```python
from build123d import *

# Parameters (mm, degrees)
F3_R = 0.99999


# Not quite as in the source:
# - a fillet or chamfer that OpenCascade refuses, or shapes differently, is made with other operations: its cross-section is extruded or revolved along the edge and cut away or added
# - a fillet or chamfer is up to 0.001 mm smaller than in the source, because OpenCascade refuses the exact size


with BuildPart() as f1:
    # F0 (on Right) → F1 (revolve)
    with BuildSketch(Plane.YZ):
        Polygon((-47.0208749175, 2.497), (-35.0208749175, 2.497), (-35.0208749175, 4.55), (-41.0208749175, 4.55), (-41.0208749175, 7.5), (-42.0208749175, 7.5), (-43.0208749175, 4.55), (-43.5208749175, 4.55), (-44.0208749175, 4.55), (-45.0208749175, 7.5), (-46.0208749175, 7.5), (-46.0208749175, 4.55), (-46.0208749175, 3.497), (-47.0208749175, 3.497), align=None)
    revolve(axis=Axis((0, -14.7727020085, 0), (0, 1, 0)))

    # F2: fillet of radius 5 on 1 edges, made by hand

    # F2_s1 → F2_t2 (revolve)
    with BuildSketch(Plane.YZ):
        with BuildLine():
            ThreePointArc((-36.460447306, 4.55), (-39.1761424288, 5.3517860941), (-41.0208749175, 7.5))
            Line((-41.0208749175, 7.5), (-41.1120834697, 7.459))
            ThreePointArc((-41.1120834697, 7.459), (-41.1208749175, 6.025), (-41.1208749175, 4.55))
            Line((-41.1208749175, 4.55), (-41.0208749175, 4.45))
            Line((-41.0208749175, 4.45), (-36.460447306, 4.45))
            Line((-36.460447306, 4.45), (-36.460447306, 4.55))
        make_face()
    revolve(axis=Axis((0, -41.0208749175, 0), (0, 1, 0)))

    # F3 (radius 1 in the source; OpenCascade refuses exactly that, so slightly less here)
    f3_edges = [f1.edges().sort_by_distance(p)[0] for p in [
        (0, -46.020875, -3.497),
    ]]
    fillet(f3_edges, radius=F3_R)


solid = f1.part
```
Model file for the job. Use its own axes, mm. A direction names the side the tool comes from. Round coordinates to 2 decimals unless told otherwise and drop trailing zeros. Write each loop counter-clockwise with the first axis right and the second up, starting at its lowest first coordinate (ties: lowest second). Pieces come first, ordered by that corner, then holes. Notation, with made-up numbers: (-38.75, 13) - (-4.75, 13) arc R25 ccw to (-4.75, 41) - close; hole circle Ø11 at (29, 16). An arc over 180 degrees is marked (long way). Use CSV: the item, a comma, the result in double quotes. Start each with the question number.
Item 1: Pin check, flat tips, straight feed: P1, Ø5, axis at x = 3, y = -41.5, coming from the -Z side; P2, Ø4, axis at x = -1, y = -38, coming from the +Z side; P3, Ø4, axis at x = -0.5, y = -41, coming from the +Z side. Stop position of each tip, or through.
Item 2: Tool access for faces 1 (the face through (-5, -46.021, 0)), 2 (the face through (-4.44, -43.53, -0.99)), 3 (the face through (-4.44, -35.75, -0.99)): list every direction of +Z, -Z, +X, -X, +Y, -Y with a clear straight run to the whole face (end or side of a thin tool).
Item 3: Drill centre lines: L1, parallel to X at y = -43.5, z = 0; L2, parallel to X at y = -41.75, z = 0; L3, parallel to X at y = -45.5, z = -6. Where is each one in solid material? Low to high. Write a range as [from, to].
Item 4: Band-saw the part on C-C (y = -41.75). Write the cut outline in (x, z).
Item 5: Band-saw the part on D-D (y = -36). Write the cut outline in (x, z), and give its area (3 significant figures).
Item 6: Two-plate mould, pull along Y, no slides. Class faces 4 (the face through (4.694, -44.083, -0.616)), 5 (the face through (-2, -47.021, 2)), 6 (the face through (1.41, -42.97, 4.48)), 7 (the face through (-2.438, -40.937, -0.541)): released by +Y, released by -Y, zero draft, split by the parting line, or undercut.
Checked values:
1,P1,"stops at z = -7.48"
1,P2,"stops at z = 5.96"
1,P3,"stops at z = 7.5"
2,face 1,"-Y"
2,face 2,"none"
2,face 3,"+Y"
3,L1,"x = [-4.55, -2.5], [2.5, 4.55]"
3,L2,"x = [-7.5, -2.5], [2.5, 7.5]"
3,L3,"x = [-4.5, 4.5]"
4,outline,"circle Ø15 at (0, 0); hole circle Ø4.99 at (0, 0)"
5,outline,"circle Ø9.1 at (0, 0); hole circle Ø4.99 at (0, 0)"
5,area,"45.5 mm²"
6,face 4,"undercut"
6,face 5,"released by -Y"
6,face 6,"undercut"
6,face 7,"zero draft"
